Work out the finished part from the listing and answer in its coordinate system (mm). A direction names the side the tool comes from. Coordinates: 2 decimals unless noted, no trailing zeros. Order: outer loops, then holes, each group sorted by start corner. A loop starts at its lowest first (then second) coordinate and runs counter-clockwise, first axis right, second up. Notation, with made-up numbers: M 40.5,61 L 99.5,61 A23 ccw 99.5,74 Z; hole C 34.5,29 d4. An arc over 180 degrees is marked long. Answer in a Markdown table with one row per item. Add a question column.
Item 1: Flat-ended cylindrical pins translate along their axes: pin 1 Ø8 at (x, z) = (5, 4.5) entering from +Y; pin 2 Ø3 at (y, z) = (77, 6.5) entering from -X; pin 3 Ø1 at (x, y) = (2, 27.5) entering from +Z; pin 4 Ø1.8 at (x, z) = (0, 7.5) entering from +Y. Find the tip coordinate at first contact, or state that the pin passes through.
Item 2: Which of the six approach directions +Z, -Z, +X, -X, +Y, -Y give full straight-line access (tool end or side, diameter ignored) to faces 4 (the face through (-5.78, 35.5, -7.54)), 5 (the face through (0, 69, 7))?
Item 3: The part is cut by section A-A (z = 0). Write down the section's boundary in (x, y).
Item 4: The part is cut by section D-D (z = -7.25). Write down the section's boundary in (x, y), then the cut area to 3 significant figures.
Item 5: The part is cut by section C-C (x = -4.25). Write down the section's boundary in (y, z), then the cut area to 3 significant figures.
Item 6: The mould has two halves that part along Z. Classify faces 1 (the face through (-6.51, 70.52, -0.13)), 2 (the face through (-4.88, 73.97, -1.08)), 3 (the face through (0, 0, 0)): released by +Z, released by -Z, zero draft, split by the parting line, or undercut.
Item 7: Consider line 1 (X direction, y = 71, z = 0); line 2 (Y direction, x = 1.75, z = 8); line 3 (Y direction, x = -1.75, z = -3.75). Determine where each line is inside the solid, lowest interval first. Write a range as from..to.
Item 8: The part is cut by section B-B (y = 77). Write down the section's boundary in (x, z).
from build123d import *

# Parameters (mm, degrees)
SKETCH_1_R          = 9.5
EXTRUDE_1_DEPTH     = 72
SKETCH_2_R          = 5
EXTRUDE_2_DEPTH     = 4
SKETCH_3_R          = 2
EXTRUDE_3_DEPTH     = 11
SKETCH_4_R          = 1
CUT_EXTRUDE_1_DEPTH = 3


with BuildPart() as part:
    # 草图1 → 凸台-拉伸1 (new body)
    with BuildSketch(Plane(origin=(0, 0, 0), x_dir=(1, 0, 0), z_dir=(0, 1, 0))):
        with Locations(Location((0, 0, 0), (0, 0, 270))):
            Circle(SKETCH_1_R)
    extrude(amount=EXTRUDE_1_DEPTH)

    # 草图2 → 凸台-拉伸2 (add)
    with BuildSketch(Plane(origin=(0, 72, 0), x_dir=(1, 0, 0), z_dir=(0, 1, 0))):
        with Locations(Location((0, 0, 0), (0, 0, 270))):
            Circle(SKETCH_2_R)
    extrude(amount=EXTRUDE_2_DEPTH)

    # 草图3 → 凸台-拉伸3 (add)
    with BuildSketch(Plane(origin=(0, 76, 0), x_dir=(1, 0, 0), z_dir=(0, 1, 0))):
        with Locations(Location((0, 0, 0), (0, 0, 270))):
            Circle(SKETCH_3_R)
    extrude(amount=EXTRUDE_3_DEPTH)

    # 草图4 → 切除-拉伸1 (cut)
    with BuildSketch(Plane(origin=(0, 72, 0), x_dir=(1, 0, 0), z_dir=(0, 1, 0))):
        with Locations(Location((7.5, 0, 0), (0, 0, 270))):
            Circle(SKETCH_4_R)
        with Locations(Location((0, 7.5, 0), (0, 0, 270))):
            Circle(SKETCH_4_R)
        with Locations(Location((0, -7.5, 0), (0, 0, 270))):
            Circle(SKETCH_4_R)
        with Locations(Location((-7.5, 0, 0), (0, 0, 270))):
            Circle(SKETCH_4_R)
    extrude(amount=-CUT_EXTRUDE_1_DEPTH, mode=Mode.SUBTRACT)


solid = part.part
Reply:
| question | item | result |
|---|---|---|
| 1 | pin 1 | stops at y = 76 |
| 1 | pin 2 | passes through |
| 1 | pin 3 | stops at z = 9.38 |
| 1 | pin 4 | stops at y = 69 |
| 2 | face 4 | +Y, -Y |
| 2 | face 5 | +Y |
| 3 | outline | M -9.5,0 L 9.5,0 L 9.5,72 L 8.5,72 L 8.5,69 L 6.5,69 L 6.5,72 L 5,72 L 5,76 L 2,76 L 2,87 L -2,87 L -2,76 L -5,76 L -5,72 L -6.5,72 L -6.5,69 L -8.5,69 L -8.5,72 L -9.5,72 Z |
| 4 | outline | M -6.14,0 L 6.14,0 L 6.14,72 L 0.97,72 L 0.97,69 L -0.97,69 L -0.97,72 L -6.14,72 Z |
| 4 | area | 878 mm2 |
| 5 | outline | M 0,-8.5 L 72,-8.5 L 72,-2.63 L 76,-2.63 L 76,2.63 L 72,2.63 L 72,8.5 L 0,8.5 Z |
| 5 | area | 1,240 mm2 |
| 6 | face 1 | undercut |
| 6 | face 2 | split by the parting line |
| 6 | face 3 | zero draft |
| 7 | line 1 | x = -9.5..-8.5, -6.5..6.5, 8.5..9.5 |
| 7 | line 2 | y = 0..72 |
| 7 | line 3 | y = 0..76 |
| 8 | outline | C 0,0 d4 |
